Verification items for this drawing (mm, ordinates from the low corner). Coordinates: 2 decimals unless noted, no trailing zeros. Order: outer loops, then holes, each group sorted by start corner. A loop starts at its lowest first (then second) coordinate and runs counter-clockwise, first axis right, second up. Notation, with made-up numbers: (20.25, -21) -> (54.25, -21) arc R31 ccw to (54.25, 13) -> close; hole circle Ø6 at (21, -27). An arc over 180 degrees is marked (long way). Put each result on its own line as item: value. Start each with the question number.
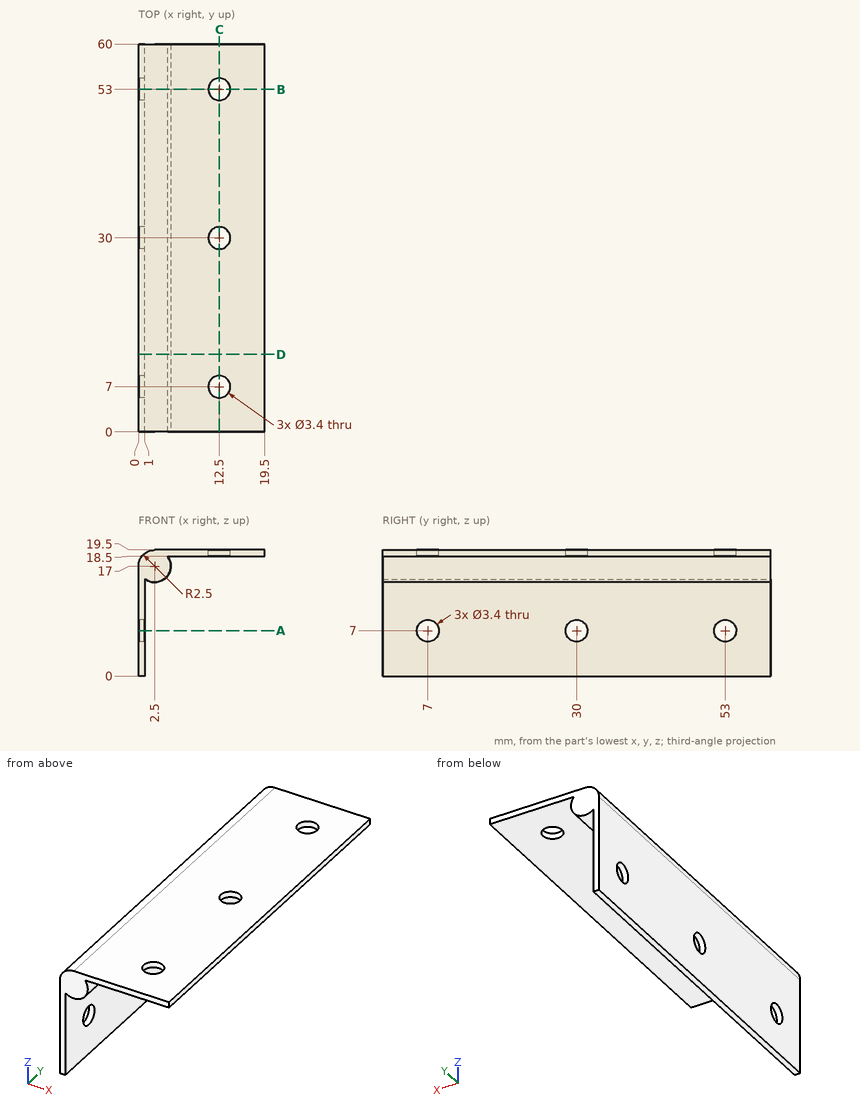
1) Scan lines: line 1 along Y through (x, z) = (0.65, 7); line 2 along Z through (x, y) = (0.5, 30); line 3 along Z through (x, y) = (0.55, 30). Record each from-to range of solid material in increasing order. Write a range as [from, to].
2) Sectioned sample at B-B (y = 53). Record the boundary of the cut face in (x, z).
3) Sectioned sample at A-A (z = 7). Record the boundary of the cut face in (x, y), plus the area to 3 significant figures.
4) Sectioned sample at C-C (x = 12.5). Record the boundary of the cut face in (y, z), plus the area to 3 significant figures.
5) Sectioned sample at D-D (y = 12). Record the boundary of the cut face in (x, z).
6) Gauge pin test, flat ends, axial feed: pin 1 (4 mm diameter, centred on y = 21.5, z = 5, fed in from +X); pin 2 (2.5 mm diameter, centred on y = 7, z = 7, fed in from +X); pin 3 (4 mm diameter, centred on x = 12.5, y = 30, fed in from -Z); pin 4 (6 mm diameter, centred on y = 34.5, z = 13.5, fed in from +X). Record the tip position at first contact, or that the pin passes through.
Entries:
1. line 1: y = [0, 5.3], [8.7, 28.3], [31.7, 51.3], [54.7, 60]
1. line 2: z = [0, 5.3], [8.7, 18.5]
1. line 3: z = [0, 5.3], [8.7, 18.56]
2. outline: (0, 0) -> (1, 0) -> (1, 5.3) -> (0, 5.3) -> close; (0, 8.7) -> (1, 8.7) -> (1, 15) arc R2.5 ccw to (4.5, 18.5) -> (10.8, 18.5) -> (10.8, 19.5) -> (2.5, 19.5) arc R2.5 ccw to (0, 17) -> close; (14.2, 18.5) -> (19.5, 18.5) -> (19.5, 19.5) -> (14.2, 19.5) -> close
3. outline: (0, 0) -> (1, 0) -> (1, 5.3) -> (0, 5.3) -> close; (0, 8.7) -> (1, 8.7) -> (1, 28.3) -> (0, 28.3) -> close; (0, 31.7) -> (1, 31.7) -> (1, 51.3) -> (0, 51.3) -> close; (0, 54.7) -> (1, 54.7) -> (1, 60) -> (0, 60) -> close
3. area: 49.8 mm2
4. outline: (0, 18.5) -> (5.3, 18.5) -> (5.3, 19.5) -> (0, 19.5) -> close; (8.7, 18.5) -> (28.3, 18.5) -> (28.3, 19.5) -> (8.7, 19.5) -> close; (31.7, 18.5) -> (51.3, 18.5) -> (51.3, 19.5) -> (31.7, 19.5) -> close; (54.7, 18.5) -> (60, 18.5) -> (60, 19.5) -> (54.7, 19.5) -> close
4. area: 49.8 mm2
5. outline: (0, 0) -> (1, 0) -> (1, 15) arc R2.5 ccw to (4.5, 18.5) -> (19.5, 18.5) -> (19.5, 19.5) -> (2.5, 19.5) arc R2.5 ccw to (0, 17) -> close
6. pin 1: stops at x = 1
6. pin 2: passes through
6. pin 3: stops at z = 18.5
6. pin 4: stops at x = 4.95
